Answer from the drawing. Dimensions are ordinates in mm from the lowest x, y and z of the part. Round coordinates to 2 decimals unless told otherwise and drop trailing zeros. Write each loop counter-clockwise with the first axis right and the second up, starting at its lowest first coordinate (ties: lowest second). Pieces come first, ordered by that corner, then holes.
1. Straight lines are drawn through the part: probe 1 along X at (y, z) = (63, 18); probe 2 along Y at (x, z) = (142, 18.25); probe 3 along X at (y, z) = (86.5, 19). For each, find the intervals that lie inside material, in ascending order.
2. Determine the mould class of the marked faces 1, 2, 3 and 4 for opening direction X: pulls with the +X half, pulls with the -X half, needs draft (parallel to the pull), parting line crosses it, or undercut.
3. Find section D-D (x = 131). Write down the section's boundary in (y, z), and give its area (3 significant figures).
4. Find section A-A (z = 14.25). Count the separate pieces of the cut face and the enclosed holes in it, and give its area (3 significant figures).
5. Find section C-C (y = 88.9). Write down the section's boundary in (x, z), and give its area (3 significant figures).
6. Find section B-B (x = 38.1). Write down the section's boundary in (y, z).
7. Flat-ended cylindrical pins translate along their axes: pin 1 Ø8 at (y, z) = (67, 6) entering from -X; pin 2 Ø8 at (x, y) = (128.5, 88.5) entering from +Z. Find the tip coordinate at first contact, or state that the pin passes through.
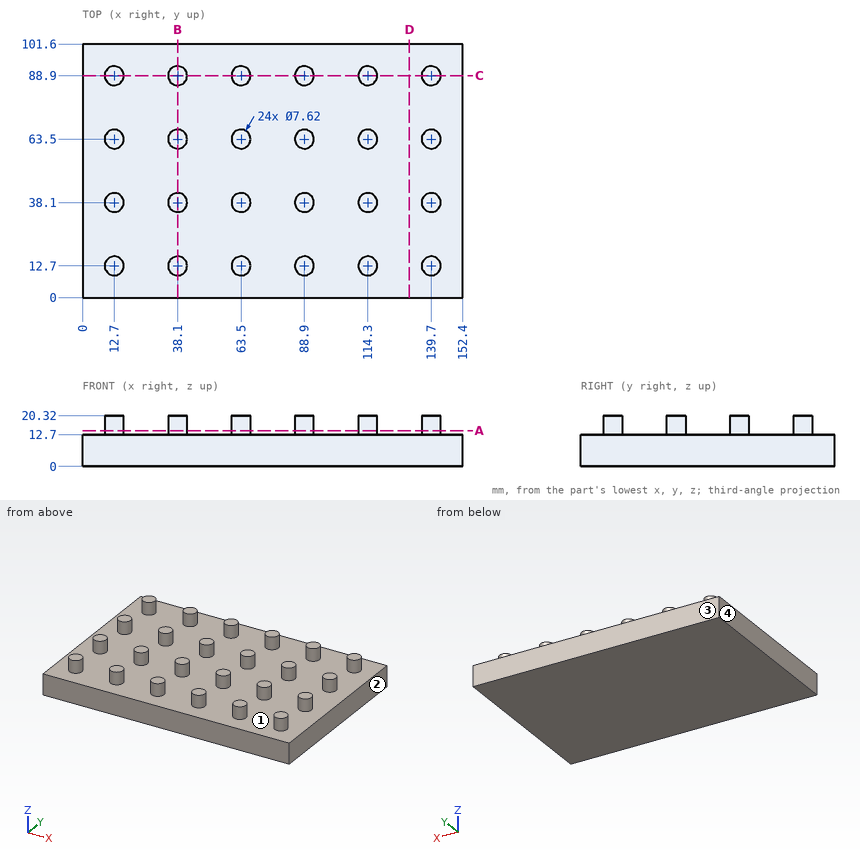
Worked answers:
1. probe 1: x = 8.92 to 16.48, 34.32 to 41.88, 59.72 to 67.28, 85.12 to 92.68, 110.52 to 118.08, 135.92 to 143.48
1. probe 2: y = 9.66 to 15.74, 35.06 to 41.14, 60.46 to 66.54, 85.86 to 91.94
1. probe 3: x = 9.74 to 15.66, 35.14 to 41.06, 60.54 to 66.46, 85.94 to 91.86, 111.34 to 117.26, 136.74 to 142.66
2. face 1: undercut
2. face 2: pulls with the +X half
2. face 3: needs draft
2. face 4: pulls with the -X half
3. outline: (0, 0) - (101.6, 0) - (101.6, 12.7) - (0, 12.7) - close
3. area: 1,290 mm2
4. separate pieces: 24
4. enclosed holes: 0
4. area: 1,090 mm2
5. outline: (0, 0) - (152.4, 0) - (152.4, 12.7) - (143.51, 12.7) - (143.51, 20.32) - (135.89, 20.32) - (135.89, 12.7) - (118.11, 12.7) - (118.11, 20.32) - (110.49, 20.32) - (110.49, 12.7) - (92.71, 12.7) - (92.71, 20.32) - (85.09, 20.32) - (85.09, 12.7) - (67.31, 12.7) - (67.31, 20.32) - (59.69, 20.32) - (59.69, 12.7) - (41.91, 12.7) - (41.91, 20.32) - (34.29, 20.32) - (34.29, 12.7) - (16.51, 12.7) - (16.51, 20.32) - (8.89, 20.32) - (8.89, 12.7) - (0, 12.7) - close
5. area: 2,280 mm2
6. outline: (0, 0) - (101.6, 0) - (101.6, 12.7) - (92.71, 12.7) - (92.71, 20.32) - (85.09, 20.32) - (85.09, 12.7) - (67.31, 12.7) - (67.31, 20.32) - (59.69, 20.32) - (59.69, 12.7) - (41.91, 12.7) - (41.91, 20.32) - (34.29, 20.32) - (34.29, 12.7) - (16.51, 12.7) - (16.51, 20.32) - (8.89, 20.32) - (8.89, 12.7) - (0, 12.7) - close
7. pin 1: stops at x = 0
7. pin 2: stops at z = 12.7
